For this review, take the finished solid that the model builds, in its own axes (mm). Face numbers are marked on the shaded views. Give positions to 0.01 mm unless a question says otherwise; leave off trailing zeros. Order: outer loops, then holes, each group sorted by start corner. A loop starts at its lowest first (then second) coordinate and runs counter-clockwise, first axis right, second up. Notation, with made-up numbers: (4, -25.5) -> (50, -25.5) arc R19 cw to (50, 9.5) -> close; hole circle Ø9 at (-11, 25). An arc over 180 degrees is marked (long way). One line per item, written item: value. Start each with the question number.
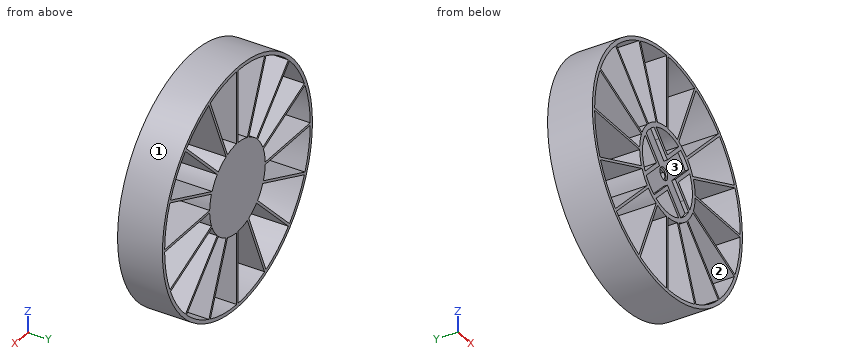
from build123d import *

# Parameters (mm, degrees)
BOSS_EXTRUDE1_OUTLINE_R = 67.5
BOSS_EXTRUDE1_DEPTH     = 25
SKETCH2_R               = 2.5
CUT_EXTRUDE2_DEPTH      = 18
SKETCH4_R               = 25
BOSS_EXTRUDE3_DEPTH     = 35
CUT_EXTRUDE4_DEPTH      = 18
CUT_EXTRUDE7_DEPTH      = 2
CUT_EXTRUDE8_DEPTH      = 20
SKETCH9_R               = 3.5
CUT_EXTRUDE9_DEPTH      = 1
CUT_EXTRUDE10_START     = -10
SKETCH10_R              = 25
CUT_EXTRUDE10_DEPTH     = 10


# Read off the part's stored shape, not the designer's step: Boss-Extrude1
with BuildPart() as part:
    # Boss-Extrude1 outline → Boss-Extrude1 (new body)
    with BuildSketch(Plane(origin=(0, 0, 0), x_dir=(1, 0, 0), z_dir=(0, 1, 0))):
        Circle(BOSS_EXTRUDE1_OUTLINE_R)
        with BuildLine():
            ThreePointArc((-13.30331837, -14.257339175), (-10.833619544, -16.21365744), (-8.081104316, -17.746711048))
            Line((-8.081104316, -17.746711048), (-25.687679516, -60.252743681))
            ThreePointArc((-25.687679516, -60.252743681), (-36.389850263, -54.461259606), (-45.836027298, -46.790048103))
            Line((-45.836027298, -46.790048103), (-13.30331837, -14.257339175))
        make_face(mode=Mode.SUBTRACT)
        with BuildLine():
            ThreePointArc((-6.834616064, -18.263023388), (-3.804261279, -19.125312968), (-0.674594581, -19.488327844))
            Line((-0.674594581, -19.488327844), (-0.674594581, -65.496526031))
            ThreePointArc((-0.674594581, -65.496526031), (-12.778416092, -64.241435866), (-24.441191264, -60.76905602))
            Line((-24.441191264, -60.76905602), (-6.834616064, -18.263023388))
        make_face(mode=Mode.SUBTRACT)
        with BuildLine():
            ThreePointArc((-17.746711048, -8.081104316), (-16.21365744, -10.833619544), (-14.257339175, -13.30331837))
            Line((-14.257339175, -13.30331837), (-46.790048103, -45.836027298))
            ThreePointArc((-46.790048103, -45.836027298), (-54.461259606, -36.389850263), (-60.252743681, -25.687679516))
            Line((-60.252743681, -25.687679516), (-17.746711048, -8.081104316))
        make_face(mode=Mode.SUBTRACT)
        with BuildLine():
            ThreePointArc((-19.488327844, -0.674594581), (-19.125312968, -3.804261279), (-18.263023388, -6.834616064))
            Line((-18.263023388, -6.834616064), (-60.76905602, -24.441191264))
            ThreePointArc((-60.76905602, -24.441191264), (-64.241435866, -12.778416092), (-65.496526031, -0.674594581))
            Line((-65.496526031, -0.674594581), (-19.488327844, -0.674594581))
        make_face(mode=Mode.SUBTRACT)
        with BuildLine():
            ThreePointArc((0.674594581, -19.488327844), (3.804261279, -19.125312968), (6.834616064, -18.263023388))
            Line((6.834616064, -18.263023388), (24.441191264, -60.76905602))
            ThreePointArc((24.441191264, -60.76905602), (12.778416092, -64.241435866), (0.674594581, -65.496526031))
            Line((0.674594581, -65.496526031), (0.674594581, -19.488327844))
        make_face(mode=Mode.SUBTRACT)
        with BuildLine():
            ThreePointArc((8.081104316, -17.746711048), (10.833619544, -16.21365744), (13.30331837, -14.257339175))
            Line((13.30331837, -14.257339175), (45.836027298, -46.790048103))
            ThreePointArc((45.836027298, -46.790048103), (36.389850263, -54.461259606), (25.687679516, -60.252743681))
            Line((25.687679516, -60.252743681), (8.081104316, -17.746711048))
        make_face(mode=Mode.SUBTRACT)
        with BuildLine():
            ThreePointArc((14.257339175, -13.30331837), (16.21365744, -10.833619544), (17.746711048, -8.081104316))
            Line((17.746711048, -8.081104316), (60.252743681, -25.687679516))
            ThreePointArc((60.252743681, -25.687679516), (54.461259606, -36.389850263), (46.790048103, -45.836027298))
            Line((46.790048103, -45.836027298), (14.257339175, -13.30331837))
        make_face(mode=Mode.SUBTRACT)
        with BuildLine():
            ThreePointArc((18.263023388, -6.834616064), (19.125312968, -3.804261279), (19.488327844, -0.674594581))
            Line((19.488327844, -0.674594581), (65.496526031, -0.674594581))
            ThreePointArc((65.496526031, -0.674594581), (64.241435866, -12.778416092), (60.76905602, -24.441191264))
            Line((60.76905602, -24.441191264), (18.263023388, -6.834616064))
        make_face(mode=Mode.SUBTRACT)
        with BuildLine():
            ThreePointArc((-18.263023388, 6.834616064), (-19.125312968, 3.804261279), (-19.488327844, 0.674594581))
            Line((-19.488327844, 0.674594581), (-65.496526031, 0.674594581))
            ThreePointArc((-65.496526031, 0.674594581), (-64.241435866, 12.778416092), (-60.76905602, 24.441191264))
            Line((-60.76905602, 24.441191264), (-18.263023388, 6.834616064))
        make_face(mode=Mode.SUBTRACT)
        with BuildLine():
            ThreePointArc((-14.257339175, 13.30331837), (-16.21365744, 10.833619544), (-17.746711048, 8.081104316))
            Line((-17.746711048, 8.081104316), (-60.252743681, 25.687679516))
            ThreePointArc((-60.252743681, 25.687679516), (-54.461259606, 36.389850263), (-46.790048103, 45.836027298))
            Line((-46.790048103, 45.836027298), (-14.257339175, 13.30331837))
        make_face(mode=Mode.SUBTRACT)
        with BuildLine():
            ThreePointArc((-8.081104316, 17.746711048), (-10.833619544, 16.21365744), (-13.30331837, 14.257339175))
            Line((-13.30331837, 14.257339175), (-45.836027298, 46.790048103))
            ThreePointArc((-45.836027298, 46.790048103), (-36.389850263, 54.461259606), (-25.687679516, 60.252743681))
            Line((-25.687679516, 60.252743681), (-8.081104316, 17.746711048))
        make_face(mode=Mode.SUBTRACT)
        with BuildLine():
            Line((-6.834616064, 18.263023388), (-24.441191264, 60.76905602))
            ThreePointArc((-24.441191264, 60.76905602), (-12.778416092, 64.241435866), (-0.674594581, 65.496526031))
            Line((-0.674594581, 65.496526031), (-0.674594581, 19.488327844))
            ThreePointArc((-0.674594581, 19.488327844), (-3.804261279, 19.125312968), (-6.834616064, 18.263023388))
        make_face(mode=Mode.SUBTRACT)
        with BuildLine():
            ThreePointArc((19.488327844, 0.674594581), (19.125312968, 3.804261279), (18.263023388, 6.834616064))
            Line((18.263023388, 6.834616064), (60.76905602, 24.441191264))
            ThreePointArc((60.76905602, 24.441191264), (64.241435866, 12.778416092), (65.496526031, 0.674594581))
            Line((65.496526031, 0.674594581), (19.488327844, 0.674594581))
        make_face(mode=Mode.SUBTRACT)
        with BuildLine():
            ThreePointArc((17.746711048, 8.081104316), (16.21365744, 10.833619544), (14.257339175, 13.30331837))
            Line((14.257339175, 13.30331837), (46.790048103, 45.836027298))
            ThreePointArc((46.790048103, 45.836027298), (54.461259606, 36.389850263), (60.252743681, 25.687679516))
            Line((60.252743681, 25.687679516), (17.746711048, 8.081104316))
        make_face(mode=Mode.SUBTRACT)
        with BuildLine():
            ThreePointArc((6.834616064, 18.263023388), (3.804261279, 19.125312968), (0.674594581, 19.488327844))
            Line((0.674594581, 19.488327844), (0.674594581, 65.496526031))
            ThreePointArc((0.674594581, 65.496526031), (12.778416092, 64.241435866), (24.441191264, 60.76905602))
            Line((24.441191264, 60.76905602), (6.834616064, 18.263023388))
        make_face(mode=Mode.SUBTRACT)
        with BuildLine():
            ThreePointArc((13.30331837, 14.257339175), (10.833619544, 16.21365744), (8.081104316, 17.746711048))
            Line((8.081104316, 17.746711048), (25.687679516, 60.252743681))
            ThreePointArc((25.687679516, 60.252743681), (36.389850263, 54.461259606), (45.836027298, 46.790048103))
            Line((45.836027298, 46.790048103), (13.30331837, 14.257339175))
        make_face(mode=Mode.SUBTRACT)
    extrude(amount=BOSS_EXTRUDE1_DEPTH)

    # Sketch2 → Cut-Extrude2 (cut)
    with BuildSketch(Plane.XZ):
        with Locations(Location((0, 0, 0), (0, 0, 270))):
            Circle(SKETCH2_R)
    extrude(amount=-CUT_EXTRUDE2_DEPTH, mode=Mode.SUBTRACT)

    # Sketch4 → Boss-Extrude3 (add)
    with BuildSketch(Plane(origin=(0, 0, 0), x_dir=(1, 0, 0), z_dir=(0, 1, 0))):
        with Locations(Location((0, 0, 0), (0, 0, 91.546244576))):
            Circle(SKETCH4_R)
    extrude(amount=BOSS_EXTRUDE3_DEPTH)

    # Sketch5 → Cut-Extrude4 (cut)
    with BuildSketch(Plane.XZ):
        with BuildLine():
            Line((-1.5, 2), (1.5, 2))
            ThreePointArc((1.5, 2), (0, -2.5), (-1.5, 2))
        make_face()
    extrude(amount=-CUT_EXTRUDE4_DEPTH, mode=Mode.SUBTRACT)

    # Sketch6 → Cut-Extrude7 (cut)
    with BuildSketch(Plane.XZ):
        with BuildLine():
            Line((-7.714466094, 14.785533906), (0, 7.071067812))
            Line((0, 7.071067812), (7.714466094, 14.785533906))
            Line((7.714466094, 14.785533906), (11.976558152, 19.047625963))
            ThreePointArc((11.976558152, 19.047625963), (15.909902577, 15.909902577), (19.047625963, 11.976558152))
            Line((19.047625963, 11.976558152), (14.785533906, 7.714466094))
            Line((14.785533906, 7.714466094), (7.071067812, 0))
            Line((7.071067812, 0), (14.785533906, -7.714466094))
            Line((14.785533906, -7.714466094), (19.047625963, -11.976558152))
            ThreePointArc((19.047625963, -11.976558152), (15.909902577, -15.909902577), (11.976558152, -19.047625963))
            Line((11.976558152, -19.047625963), (7.714466094, -14.785533906))
            Line((7.714466094, -14.785533906), (0, -7.071067812))
            Line((0, -7.071067812), (-7.714466094, -14.785533906))
            Line((-7.714466094, -14.785533906), (-11.976558152, -19.047625963))
            ThreePointArc((-11.976558152, -19.047625963), (-15.909902577, -15.909902577), (-19.047625963, -11.976558152))
            Line((-19.047625963, -11.976558152), (-14.785533906, -7.714466094))
            Line((-14.785533906, -7.714466094), (-7.071067812, 0))
            Line((-7.071067812, 0), (-14.785533906, 7.714466094))
            Line((-14.785533906, 7.714466094), (-19.047625963, 11.976558152))
            ThreePointArc((-19.047625963, 11.976558152), (-15.909902577, 15.909902577), (-11.976558152, 19.047625963))
            Line((-11.976558152, 19.047625963), (-7.714466094, 14.785533906))
        make_face()
    extrude(amount=-CUT_EXTRUDE7_DEPTH, mode=Mode.SUBTRACT)

    # Sketch7 → Cut-Extrude8 (cut)
    with BuildSketch(Plane.XZ):
        with BuildLine():
            Line((9.899494937, 0), (20.070097993, 10.170603057))
            ThreePointArc((20.070097993, 10.170603057), (22.5, 0), (20.070097993, -10.170603057))
            Line((20.070097993, -10.170603057), (9.899494937, 0))
        make_face()
        with BuildLine():
            Line((0, 9.899494937), (-10.170603057, 20.070097993))
            ThreePointArc((-10.170603057, 20.070097993), (0, 22.5), (10.170603057, 20.070097993))
            Line((10.170603057, 20.070097993), (0, 9.899494937))
        make_face()
        with BuildLine():
            Line((0, -9.899494937), (10.170603057, -20.070097993))
            ThreePointArc((10.170603057, -20.070097993), (0, -22.5), (-10.170603057, -20.070097993))
            Line((-10.170603057, -20.070097993), (0, -9.899494937))
        make_face()
        with BuildLine():
            Line((-9.899494937, 0), (-20.070097993, -10.170603057))
            ThreePointArc((-20.070097993, -10.170603057), (-22.5, 0), (-20.070097993, 10.170603057))
            Line((-20.070097993, 10.170603057), (-9.899494937, 0))
        make_face()
    extrude(amount=-CUT_EXTRUDE8_DEPTH, mode=Mode.SUBTRACT)

    # Sketch9 → Cut-Extrude9 (cut)
    with BuildSketch(Plane(origin=(0, 2, 0), x_dir=(-1, 0, 0), z_dir=(0, -1, 0))):
        with Locations(Location((0, 0, 0), (0, 0, 90))):
            Circle(SKETCH9_R)
    extrude(amount=-CUT_EXTRUDE9_DEPTH, mode=Mode.SUBTRACT)

    # Sketch10 → Cut-Extrude10 (cut)
    with BuildSketch(Plane(origin=(0, 35, 0), x_dir=(1, 0, 0), z_dir=(0, 1, 0)).offset(CUT_EXTRUDE10_START)):
        Circle(SKETCH10_R)
    extrude(amount=CUT_EXTRUDE10_DEPTH, mode=Mode.SUBTRACT)


solid = part.part
Q1. For pin 1 Ø12.5 at (x, y) = (47, 11.5) entering from +Z; pin 2 Ø4 at (y, z) = (14.5, -8) entering from -X; pin 3 Ø1 at (x, y) = (43.5, 8.5) entering from +Z; pin 4 Ø3 at (x, z) = (52, -26) entering from +Y, all flat-tipped, find the tip position at first contact; note any pin that passes through.
Q2. Mouldability with a two-part tool opening along X and no side actions: class the marked faces 1, 2 and 3 as pulls with the +X half, pulls with the -X half, needs draft (parallel to the pull), parting line crosses it, or undercut.
Q3. Take a section at C-C (y = 6). State how many separate pieces and enclosed holes the cut face has, and give its area (3 significant figures).
Q4. Take a section at A-A (z = -32). State the section outline as (x, y) points (3 decimals).
Q5. For line 1 along X through (y, z) = (7.5, 0); line 2 along X through (y, z) = (2.3, 0); line 3 along Z through (x, y) = (0, 6.5), list the stretches that pass through material, from the lowest coordinate up.
Q6. Take a section at B-B (x = 29.5). State the section outline as (y, z) points.
Answers below:
1. pin 1: stops at z = 53.81
1. pin 2: stops at x = -67.23
1. pin 3: stops at z = 52.03
1. pin 4: passes through
2. face 1: parting line crosses it
2. face 2: undercut
2. face 3: undercut
3. separate pieces: 1
3. enclosed holes: 21
3. area: 3,110 mm²
4. outline: (-59.433, 0) -> (-57.151, 0) -> (-57.151, 25) -> (-59.433, 25) -> close; (-32.954, 0) -> (-31.046, 0) -> (-31.046, 25) -> (-32.954, 25) -> close; (-13.985, 0) -> (-12.525, 0) -> (-12.525, 25) -> (-13.985, 25) -> close; (-0.675, 0) -> (0.675, 0) -> (0.675, 25) -> (-0.675, 25) -> close; (12.525, 0) -> (13.985, 0) -> (13.985, 25) -> (12.525, 25) -> close; (31.046, 0) -> (32.954, 0) -> (32.954, 25) -> (31.046, 25) -> close; (57.151, 0) -> (59.433, 0) -> (59.433, 25) -> (57.151, 25) -> close
5. line 1: x = -67.5 to -22.5, -9.9 to -2.5, 2.5 to 9.9, 22.5 to 67.5
5. line 2: x = -67.5 to -22.5, -9.9 to -3.5, 3.5 to 9.9, 22.5 to 67.5
5. line 3: z = -67.5 to -22.5, -9.9 to -2.5, 2 to 9.9, 22.5 to 67.5
6. outline: (0, -60.71) -> (25, -60.71) -> (25, -58.48) -> (0, -58.48) -> close; (0, -30.45) -> (25, -30.45) -> (25, -28.55) -> (0, -28.55) -> close; (0, -12.95) -> (25, -12.95) -> (25, -11.49) -> (0, -11.49) -> close; (0, -0.67) -> (25, -0.67) -> (25, 0.67) -> (0, 0.67) -> close; (0, 11.49) -> (25, 11.49) -> (25, 12.95) -> (0, 12.95) -> close; (0, 28.55) -> (25, 28.55) -> (25, 30.45) -> (0, 30.45) -> close; (0, 58.48) -> (25, 58.48) -> (25, 60.71) -> (0, 60.71) -> close
